from build123d import *

# Parameters (mm, degrees)
BOSS_EXTRUDE1_DEPTH = 25.4
CUT_EXTRUDE1_REACH  = 27.4
SKETCH2_R           = 3.175
SKETCH2_R_2         = 0.79375
SKETCH3_W           = 3.175
SKETCH3_H           = 1.5875
CUT_EXTRUDE2_DEPTH  = 26.4
SKETCH4_R           = 8.001
CUT_EXTRUDE3_DEPTH  = 5.08
SKETCH5_R           = 3.302
CUT_EXTRUDE4_DEPTH  = 21.32


with BuildPart() as part:
    # Sketch1 → Boss-Extrude1 (new body)
    with BuildSketch(Plane.XY):
        with BuildLine():
            Line((12.7, 50.8), (12.7, -50.8))
            ThreePointArc((12.7, -50.8), (0, -63.5), (-12.7, -50.8))
            Line((-12.7, -50.8), (-12.7, 50.8))
            ThreePointArc((-12.7, 50.8), (0, 63.5), (12.7, 50.8))
        make_face()
    extrude(amount=BOSS_EXTRUDE1_DEPTH)

    # Sketch2 → Cut-Extrude1 (cut, up to next)
    with BuildSketch(Plane.XY.offset(25.4), mode=Mode.PRIVATE) as cut_extrude1_sk1:
        with Locations((0, 50.8)):
            Circle(SKETCH2_R)
    cut_extrude1_tool1 = extrude(cut_extrude1_sk1.sketch, amount=-CUT_EXTRUDE1_REACH, mode=Mode.PRIVATE) & part.part
    add(cut_extrude1_tool1.solids().sort_by_distance((0, 50.8, 25.4))[0], mode=Mode.SUBTRACT)
    # Sketch2 → Cut-Extrude1 (cut, up to next)
    with BuildSketch(Plane.XY.offset(25.4), mode=Mode.PRIVATE) as cut_extrude1_sk2:
        with Locations((-4.939140867, 55.739140867)):
            Circle(SKETCH2_R_2)
    cut_extrude1_tool2 = extrude(cut_extrude1_sk2.sketch, amount=-CUT_EXTRUDE1_REACH, mode=Mode.PRIVATE) & part.part
    add(cut_extrude1_tool2.solids().sort_by_distance((-4.939141, 55.739141, 25.4))[0], mode=Mode.SUBTRACT)
    # Sketch2 → Cut-Extrude1 (cut, up to next)
    with BuildSketch(Plane.XY.offset(25.4), mode=Mode.PRIVATE) as cut_extrude1_sk3:
        with Locations((-4.939140867, 45.860859133)):
            Circle(SKETCH2_R_2)
    cut_extrude1_tool3 = extrude(cut_extrude1_sk3.sketch, amount=-CUT_EXTRUDE1_REACH, mode=Mode.PRIVATE) & part.part
    add(cut_extrude1_tool3.solids().sort_by_distance((-4.939141, 45.860859, 25.4))[0], mode=Mode.SUBTRACT)
    # Sketch2 → Cut-Extrude1 (cut, up to next)
    with BuildSketch(Plane.XY.offset(25.4), mode=Mode.PRIVATE) as cut_extrude1_sk4:
        with Locations((4.939140867, 55.739140867)):
            Circle(SKETCH2_R_2)
    cut_extrude1_tool4 = extrude(cut_extrude1_sk4.sketch, amount=-CUT_EXTRUDE1_REACH, mode=Mode.PRIVATE) & part.part
    add(cut_extrude1_tool4.solids().sort_by_distance((4.939141, 55.739141, 25.4))[0], mode=Mode.SUBTRACT)
    # Sketch2 → Cut-Extrude1 (cut, up to next)
    with BuildSketch(Plane.XY.offset(25.4), mode=Mode.PRIVATE) as cut_extrude1_sk5:
        with Locations((4.939140867, 45.860859133)):
            Circle(SKETCH2_R_2)
    cut_extrude1_tool5 = extrude(cut_extrude1_sk5.sketch, amount=-CUT_EXTRUDE1_REACH, mode=Mode.PRIVATE) & part.part
    add(cut_extrude1_tool5.solids().sort_by_distance((4.939141, 45.860859, 25.4))[0], mode=Mode.SUBTRACT)

    # Sketch3 → Cut-Extrude2 (cut, through all)
    with BuildSketch(Plane.XY.offset(25.4)):
        with Locations((0, 54.343380657)):
            Rectangle(SKETCH3_W, SKETCH3_H)
    extrude(amount=-CUT_EXTRUDE2_DEPTH, mode=Mode.SUBTRACT)

    # Sketch4 → Cut-Extrude3 (cut)
    with BuildSketch(Plane.XY.offset(25.4)):
        with Locations((0, -50.8)):
            Circle(SKETCH4_R)
    cut_extrude3 = extrude(amount=-CUT_EXTRUDE3_DEPTH, mode=Mode.SUBTRACT)

    # Mirror1: Cut-Extrude3 across plane
    add(cut_extrude3.mirror(Plane.XY.offset(12.7)), mode=Mode.SUBTRACT)

    # Sketch5 → Cut-Extrude4 (cut, through all)
    with BuildSketch(Plane.XY.offset(20.32)):
        with Locations((0, -50.8)):
            Circle(SKETCH5_R)
    extrude(amount=-CUT_EXTRUDE4_DEPTH, mode=Mode.SUBTRACT)


solid = part.part
Check sheet for the modelled part. Datum: model origin and axes. Units: mm. A direction names the side the tool comes from. Round coordinates to 2 decimals unless told otherwise and drop trailing zeros. Loops run counter-clockwise (first coordinate to the right, second up) from the corner with the lowest first, then second, coordinate; pieces in that order, holes last. Notation, with made-up numbers: (44.25, 22) - (101.25, 22) arc R15 ccw to (101.25, 26) - close; hole circle Ø10 at (43, -2.75). An arc over 180 degrees is marked (long way). Answer as CSV lines item,"result". Start each with the question number.
Item 1: Release check for a two-part mould opening along Y. For faces 5 (the flat face through (3.4, -52.5, 5.08)), 6 (the flat face through (12.7, 1, 13)), 7 (the cylindrical face through (-0.279, 63.497, 12.522)) record: +Y half, -Y half, draft (parallel to the pull), parting line (faces both ways), or undercut.
Item 2: Depth check by flat-ended pin: P1, Ø6, axis at x = 0, y = -50.8, coming from the +Z side; P2, Ø6, axis at x = 9, z = 21.5, coming from the +Y side; P3, Ø1, axis at x = 1, z = 10.5, coming from the -Y side; P4, Ø14.5, axis at x = 0, y = -50.8, coming from the -Z side. Enter the tip coordinate at first touch or a pass-through.
Item 3: Scan lines: line 1 (Y direction, x = 0, z = 8.5) (3 decimals); line 2 (Y direction, x = 0, z = 22.15) (3 decimals); line 3 (Y direction, x = -3.75, z = 22.75). Record each from-to range of solid material in increasing order. Write a range as [from, to].
Item 4: Section check B-B (z = 12.5). Count the separate pieces of the cut face and the enclosed holes in it, and give its area (3 significant figures).
Item 5: Set-up check for faces 1 (the flat face through (0, 1, 25.4)), 2 (the flat face through (0, 55.137, 13)), 3 (the cylindrical face through (-1.73, -58.61, 2.5)), 4 (the flat face through (3.4, -52.5, 20.32)): record each of +Z, -Z, +X, -X, +Y, -Y from which the full face is reachable in a straight line by a thin tool's end or side.
Item 6: Section check A-A (x = 0). Record the boundary of the cut face in (y, z) (3 decimals), and give its area (3 significant figures).
Report:
1,face 5,"undercut"
1,face 6,"draft"
1,face 7,"+Y half"
2,P1,"passes through"
2,P2,"stops at y = 61.99"
2,P3,"stops at y = -63.49"
2,P4,"stops at z = 5.08"
3,line 1,"y = [-63.5, -54.102], [-47.498, 47.625], [55.137, 63.5]"
3,line 2,"y = [-63.5, -58.801], [-42.799, 47.625], [55.137, 63.5]"
3,line 3,"y = [-62.93, -57.87], [-43.73, 62.93]"
4,separate pieces,"1"
4,enclosed holes,"6"
4,area,"3,010 mm2"
5,face 1,"+Z, +X, -X, +Y, -Y"
5,face 2,"+Z, -Z"
5,face 3,"-Z"
5,face 4,"+Z"
6,outline,"(-63.5, 0) - (-58.801, 0) - (-58.801, 5.08) - (-54.102, 5.08) - (-54.102, 20.32) - (-58.801, 20.32) - (-58.801, 25.4) - (-63.5, 25.4) - close; (-47.498, 5.08) - (-42.799, 5.08) - (-42.799, 0) - (47.625, 0) - (47.625, 25.4) - (-42.799, 25.4) - (-42.799, 20.32) - (-47.498, 20.32) - close; (55.137, 0) - (63.5, 0) - (63.5, 25.4) - (55.137, 25.4) - close"
6,area,"2,770 mm2"
